Verification items for this drawing (mm, ordinates from the low corner). A direction names the side the tool comes from. Coordinates: 2 decimals unless noted, no trailing zeros. Write each loop counter-clockwise with the first axis right and the second up, starting at its lowest first coordinate (ties: lowest second). Pieces come first, ordered by that corner, then holes. Notation, with made-up numbers: (-34.75, -2) -> (22.25, -2) arc R10 cw to (22.25, 15) -> close; hole circle Ø7 at (-30, -12). An arc over 180 degrees is marked (long way). Answer as CSV lines item,"result".
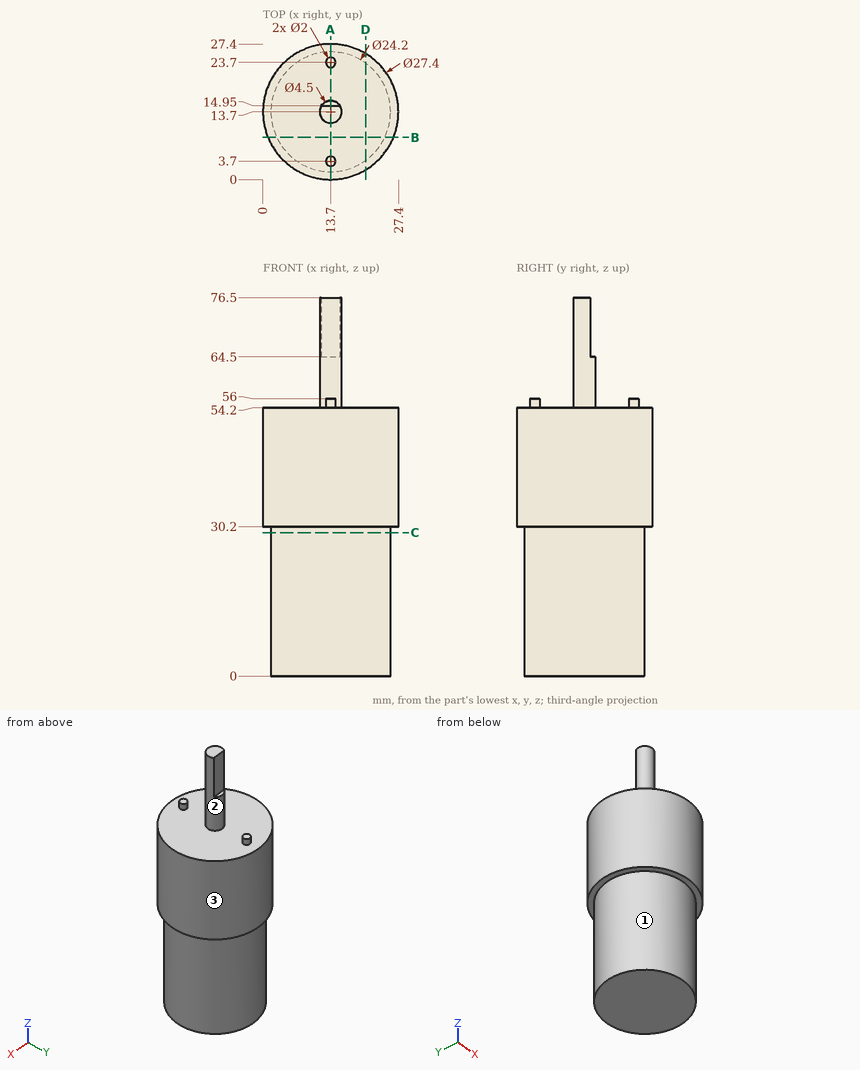
Item 1: Set-up check for the marked faces 1, 2 and 3: record each of +Z, -Z, +X, -X, +Y, -Y from which the full face is reachable in a straight line by a thin tool's end or side.
Responses:
face 1,"-Z"
face 2,"+Z"
face 3,"+Z, -Z"
Item 2: Cross-section at D-D, the plane x = 20.75. Record the cut outline in (y, z), plus the area to 3 significant figures.
Responses:
outline,"(1.95, 30.2) -> (3.87, 30.2) -> (3.87, 0) -> (23.53, 0) -> (23.53, 30.2) -> (25.45, 30.2) -> (25.45, 54.2) -> (1.95, 54.2) -> close"
area,"1,160 mm2"
Item 3: Cross-section at B-B, the plane y = 8.5. Record the cut outline in (x, z).
Responses:
outline,"(1.03, 30.2) -> (2.77, 30.2) -> (2.77, 0) -> (24.63, 0) -> (24.63, 30.2) -> (26.37, 30.2) -> (26.37, 54.2) -> (1.03, 54.2) -> close"
Item 4: Depth check by flat-ended pin: pin 1 Ø3 at (x, z) = (11, 61.5) entering from -Y; pin 2 Ø1 at (y, z) = (14.5, 48) entering from -X; pin 3 Ø6 at (x, z) = (12.5, 63) entering from -Y; pin 4 Ø13.5 at (x, y) = (7, 10.5) entering from -Z. Enter the tip coordinate at first touch or a pass-through.
Responses:
pin 1,"stops at y = 11.8"
pin 2,"stops at x = 0"
pin 3,"stops at y = 11.45"
pin 4,"stops at z = 0"
Item 5: Cross-section at C-C, the plane z = 29. Record the cut outline in (x, y), plus the area to 3 significant figures.
Responses:
outline,"circle Ø24.2 at (13.7, 13.7)"
area,"460 mm2"
Item 6: Thickness scan on probe 1 along Z at (x, y) = (19, 13.5); probe 2 along Y at (x, z) = (13.75, 41); probe 3 along X at (y, z) = (1.75, 36). Record the ranges inside material, lowest first.
Responses:
probe 1,"z = 0 to 54.2"
probe 2,"y = 0 to 27.4"
probe 3,"x = 7 to 20.4"
Item 7: Cross-section at A-A, the plane x = 13.7. Record the cut outline in (y, z), plus the area to 3 significant figures.
Responses:
outline,"(0, 30.2) -> (1.6, 30.2) -> (1.6, 0) -> (25.8, 0) -> (25.8, 30.2) -> (27.4, 30.2) -> (27.4, 54.2) -> (24.7, 54.2) -> (24.7, 56) -> (22.7, 56) -> (22.7, 54.2) -> (15.95, 54.2) -> (15.95, 64.5) -> (14.95, 64.5) -> (14.95, 76.5) -> (11.45, 76.5) -> (11.45, 54.2) -> (4.7, 54.2) -> (4.7, 56) -> (2.7, 56) -> (2.7, 54.2) -> (0, 54.2) -> close"
area,"1,480 mm2"
